Source: CAD feature listing. Evaluate the final solid. Frame: model axes, mm. Face numbers are marked on the shaded views. A direction names the side the tool comes from. Coordinates: 2 decimals unless noted, no trailing zeros. Order: outer loops, then holes, each group sorted by start corner. A loop starts at its lowest first (then second) coordinate and runs counter-clockwise, first axis right, second up. Notation, with made-up numbers: (55, 83) - (90, 83) arc R16 cw to (90, 113) - close; hole circle Ø1 at (-34, 20.5). An arc over 180 degrees is marked (long way). One line per question, with ' | ' between items. Start each with the question number.
(1) Section B-B (z = -20). Return the cut outline in (x, y), then the cut area to 3 significant figures.
(2) Section A-A (x = 38). Return the cut outline in (y, z), then the cut area to 3 significant figures.
(3) Access query for the marked faces 4 and 5. Directions: +Z, -Z, +X, -X, +Y, -Y. A direction counts if a zero-diameter tool reaches every point of the face in a straight line with its end or side. Return the directions, or none.
(4) Contact query for flat-ended pins moving along their axis: P1, Ø3.5, axis at x = -38, z = -20, coming from the +Y side; P2, Ø2, axis at x = 17, y = 45.5, coming from the +Z side; P3, Ø2, axis at y = 35.5, z = 9.5, coming from the +X side. Output: stop coordinate, or through.
(5) Draft query along X for the marked faces 1, 2 and 3. Return one class per face: +X half, -X half, draft (parallel to the pull), parting line (faces both ways), or undercut.
(6) Section D-D (z = 7.5). Return the cut outline in (x, y).
(7) Section C-C (x = 6.5). Return the cut outline in (y, z), then the cut area to 3 significant figures.
(8) Line query: line 1 along Z through (x, y) = (38, 4); line 2 along X through (y, z) = (2, -20); line 3 along Z through (x, y) = (0, 45). Output: solid intervals per line, ascending.
from build123d import *

# Parameters (mm, degrees)
IZIM1_R                     = 30
Y_KSEKLIK_EKSTR_ZYON1_DEPTH = 65
IZIM2_R                     = 26
KES_EKSTR_ZYON1_DEPTH       = 62
Y_KSEKLIK_EKSTR_ZYON4_START = 10
IZIM3_R                     = 3
Y_KSEKLIK_EKSTR_ZYON4_DEPTH = 52
IZIM4_R                     = 2
KES_EKSTR_ZYON2_DEPTH       = 52
IZIM5_W                     = 90
IZIM5_H                     = 60
Y_KSEKLIK_EKSTR_ZYON5_DEPTH = 7
IZIM6_R                     = 1.5
KES_EKSTR_ZYON3_DEPTH       = 10
IZIM7_R                     = 1.5
KES_EKSTR_ZYON4_DEPTH       = 10


with BuildPart() as part:
    # Çizim1 → Yükseklik-Ekstrüzyon1 (new body)
    with BuildSketch(Plane(origin=(0, 0, 0), x_dir=(1, 0, 0), z_dir=(0, 1, 0))):
        Circle(IZIM1_R)
    extrude(amount=Y_KSEKLIK_EKSTR_ZYON1_DEPTH)

    # Çizim2 → Kes-Ekstrüzyon1 (cut)
    with BuildSketch(Plane(origin=(0, 65, 0), x_dir=(1, 0, 0), z_dir=(0, 1, 0))):
        Circle(IZIM2_R)
    extrude(amount=-KES_EKSTR_ZYON1_DEPTH, mode=Mode.SUBTRACT)

    # Çizim3 → Yükseklik-Ekstrüzyon4 (add)
    with BuildSketch(Plane(origin=(0, 3, 0), x_dir=(1, 0, 0), z_dir=(0, 1, 0)).offset(Y_KSEKLIK_EKSTR_ZYON4_START)):
        with Locations((-22.975460117, -1.129367831)):
            Circle(IZIM3_R)
    extrude(amount=Y_KSEKLIK_EKSTR_ZYON4_DEPTH)

    # Çizim4 → Kes-Ekstrüzyon2 (cut)
    with BuildSketch(Plane(origin=(0, 65, 0), x_dir=(1, 0, 0), z_dir=(0, 1, 0))):
        with Locations((-22.975460117, -1.129367831)):
            Circle(IZIM4_R)
    extrude(amount=-KES_EKSTR_ZYON2_DEPTH, mode=Mode.SUBTRACT)

    # Çizim5 → Yükseklik-Ekstrüzyon5 (add)
    with BuildSketch(Plane.XZ):
        Rectangle(IZIM5_W, IZIM5_H)
    extrude(amount=-Y_KSEKLIK_EKSTR_ZYON5_DEPTH)

    # Çizim6 → Kes-Ekstrüzyon3 (cut)
    with BuildSketch(Plane(origin=(0, 7, 0), x_dir=(1, 0, 0), z_dir=(0, 1, 0))):
        with Locations((38, 0)):
            Circle(IZIM6_R)
        with Locations((-38, 0)):
            Circle(IZIM6_R)
    extrude(amount=-KES_EKSTR_ZYON3_DEPTH, mode=Mode.SUBTRACT)

    # Çizim7 → Kes-Ekstrüzyon4 (cut)
    with BuildSketch(Plane(origin=(0, 7, 0), x_dir=(1, 0, 0), z_dir=(0, 1, 0))):
        with Locations((-38, 20)):
            Circle(IZIM7_R)
        with Locations((-38, -20)):
            Circle(IZIM7_R)
        with Locations((38, -20)):
            Circle(IZIM7_R)
        with Locations((38, 20)):
            Circle(IZIM7_R)
    extrude(amount=-KES_EKSTR_ZYON4_DEPTH, mode=Mode.SUBTRACT)


solid = part.part
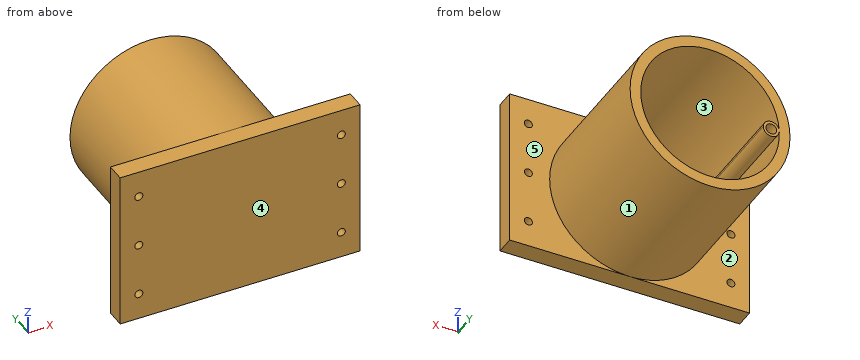
Response values:
1) outline: (-45, 0) - (-39.5, 0) - (-39.5, 7) - (-45, 7) - close; (-36.5, 0) - (36.5, 0) - (36.5, 7) - (22.36, 7) - (22.36, 65) - (16.61, 65) - (16.61, 7) - (-16.61, 7) - (-16.61, 65) - (-22.36, 65) - (-22.36, 7) - (-36.5, 7) - close; (39.5, 0) - (45, 0) - (45, 7) - (39.5, 7) - close | area: 1,250 mm²
2) outline: (0, -30) - (7, -30) - (7, -21.5) - (0, -21.5) - close; (0, -18.5) - (7, -18.5) - (7, -1.5) - (0, -1.5) - close; (0, 1.5) - (7, 1.5) - (7, 18.5) - (0, 18.5) - close; (0, 21.5) - (7, 21.5) - (7, 30) - (0, 30) - close | area: 357 mm²
3) face 4: +Z, -Z, +X, -X, -Y | face 5: +X, +Y
4) P1: stops at y = 7 | P2: stops at z = 25.38 | P3: stops at x = 28.77
5) face 1: parting line | face 2: draft | face 3: undercut
6) outline: (-45, 0) - (45, 0) - (45, 7) - (29.05, 7) - (29.05, 65) - (24.89, 65) - (24.89, 7) - (-24.89, 7) - (-24.89, 65) - (-29.05, 65) - (-29.05, 7) - (-45, 7) - close
7) outline: (0, -30) - (7, -30) - (7, -29.29) - (65, -29.29) - (65, -25.17) - (7, -25.17) - (7, 25.17) - (65, 25.17) - (65, 29.29) - (7, 29.29) - (7, 30) - (0, 30) - close | area: 897 mm²
8) line 1: z = -30 to -21.5, -18.5 to -1.5, 1.5 to 18.5, 21.5 to 30 | line 2: x = -45 to -39.5, -36.5 to 36.5, 39.5 to 45 | line 3: z = -30 to -26, 26 to 30
